Build history of the part. All positions in model axes, mm. A direction names the side the tool comes from. Round coordinates to 2 decimals unless told otherwise and drop trailing zeros. Write each loop counter-clockwise with the first axis right and the second up, starting at its lowest first coordinate (ties: lowest second). Pieces come first, ordered by that corner, then holes. Notation, with made-up numbers: (20.25, 88) -> (65.25, 88) arc R28 ccw to (65.25, 111) -> close; hole circle Ø4 at (74, 60). An arc over 180 degrees is marked (long way). Return JSON: item names as keys, results as strings.
Autodesk Inventor part; units mm, degrees
ref_plane "YZ Plane" through (0, 0, 0) normal (1, 0, 0) x (0, 1, 0)
ref_plane "XZ Plane" through (0, 0, 0) normal (0, 1, 0) x (-1, 0, 0)
ref_plane "XY Plane" through (0, 0, 0) normal (0, 0, 1) x (1, 0, 0)
sketch "Szkic1" plane through (0, 0, 0) normal (1, 0, 0) x (0, 1, 0)
  arc A0 (-13.3906, 4.8738) -> (13.3906, 4.8738) centre (0, 0) ccw
  arc A1 (-16.7323, 0.7692) -> (16.7323, 0.7692) centre (0, 0) ccw
  line L0 (13.3906, 4.8738) -> (15.7399, 5.7288)
  line L1 (0, 0) -> (16.75, 0) construction
  line L2 (0, 0) -> (0, 14)
  line L3 (-13.3906, 4.8738) -> (-15.7399, 5.7288)
  line L4 (0, 14) -> (0, 16.75)
  line L5 (12.5, 24) -> (22.5, 24)
  line L6 (-12.5, 24) -> (-22.5, 24)
  line L7 (22.2845, 26.5) -> (12.5, 26.5)
  line L8 (12.5, 26.5) -> (12.5, 24)
  line L9 (22.2845, 26.5) -> (22.2845, 28)
  line L10 (22.2845, 28) -> (12.5, 28)
  line L11 (12.5, 28) -> (12.5, 30.5)
  line L12 (12.5, 30.5) -> (22.2845, 30.5)
  line L13 (-22.5, 24) -> (-12.5, 24)
  line L14 (-12.5, 24) -> (-12.5, 26.5)
  line L15 (-12.5, 26.5) -> (-22.5, 26.5)
  line L16 (-22.5, 26.5) -> (-22.5, 28)
  line L17 (-22.5, 28) -> (-12.5, 28)
  line L18 (-12.5, 28) -> (-12.5, 30.5)
  line L19 (-12.5, 30.5) -> (-22.5, 30.5)
  line L20 (22.5, 24) -> (22.5, 8.1893)
  line L21 (22.5, 8.1893) -> (15.7399, 5.7288)
  line L22 (-22.5, 24) -> (-22.5, 8.1893)
  line L23 (-22.5, 8.1893) -> (-15.7399, 5.7288)
  line L24 (-22.5, 30.5) -> (-27.5, 30.5)
  line L25 (-27.5, 30.5) -> (-27.5, 10.0092)
  line L26 (22.2845, 30.5) -> (27.2845, 30.5)
  line L27 (27.2845, 30.5) -> (27.2845, 10.0135)
  line L28 (20.83, 2.2606) -> (27.2845, 4.6099)
  line L29 (27.2845, 4.6099) -> (27.2845, 10.0135)
  line L30 (20.83, 2.2606) -> (16.7323, 0.7692)
  line L31 (-20.83, 2.2606) -> (-16.7323, 0.7692)
  line L32 (-20.83, 2.2606) -> (-27.5, 4.6099)
  line L33 (-27.5, 4.6099) -> (-27.5, 10.0092)
  dimension "d26" = 5
  dimension "d27" = 5
extrude "Wyciągnięcie proste1" add sketch "Szkic1" along normal blind 75
sketch "Szkic2" plane through (0, 12.5, 30.5) normal (0, 0, 1) x (1, 0, 0)
  line L0 (0, 14.7845) -> (75, 14.7845)
  line L1 (0, 14.7845) -> (9, 14.7845)
  line L2 (75, -40) -> (75, -33.33)
  line L3 (75, -40) -> (66, -40)
  line L4 (9, 14.7845) -> (66, 14.7845)
  line L5 (66, 14.7845) -> (66, -40)
  line L6 (66, -40) -> (9, -40)
  line L7 (9, -40) -> (9, 14.7845)
  point P0 (0, -12.5)
  dimension "d32" = 9
  dimension "d33" = 9
extrude "Wyciągnięcie proste2" cut sketch "Szkic2" against normal blind 10.5
sketch "Szkic3" plane through (0, 12.5, 30.5) normal (0, 0, 1) x (1, 0, 0)
  line L0 (0, 0) -> (0, 9.7845)
  line L1 (5, 0) -> (0, 0)
  circle A0 centre (5, 5) radius 1.75
  line L2 (0, -25) -> (9, -25)
  line L3 (5, -25) -> (0, -25)
  circle A1 centre (5, -30) radius 1.75
  line L4 (66, -25) -> (75, -25)
  circle A2 centre (70, -30) radius 1.75
  circle A3 centre (70.1447, 5) radius 1.75
  point P0 (0, -12.5)
  dimension "d39" = 3.5
  dimension "d42" = 3.5
  dimension "d46" = 3.5
  dimension "d48" = 3.5
extrude "Wyciągnięcie proste3" cut sketch "Szkic3" against normal blind 10.5
properties part number "obejmadrążka"
Q1. Pin check, flat tips, straight feed: pin 1 Ø10 at (x, y) = (70, 18) entering from -Z; pin 2 Ø4 at (x, y) = (70.14, 17.5) entering from -Z; pin 3 Ø12 at (x, y) = (54, 7.5) entering from +Z; pin 4 Ø4 at (y, z) = (19.5, 13) entering from +X. Stop position of each tip, or through.
Verdict:
{"pin 1": "stops at z = -10.56", "pin 2": "stops at z = -6.35", "pin 3": "stops at z = 4.91", "pin 4": "passes through"}
Q2. Saw through at D-D on x = 5. Count the separate pieces of the cut face and the enclosed holes in it, then the cut area to 3 significant figures.
Verdict:
{"separate pieces": "5", "enclosed holes": "0", "area": "541 mm²"}
Q3. Wall check: L1, parallel to Y at x = 5, z = 24.9; L2, parallel to Y at x = 40.5, z = 15.5; L3, parallel to Y at x = 49, z = 0. Give the ranges that are in metal, low to high.
Verdict:
{"L1": "y = -27.5 to -19.25, -15.75 to -12.5, 12.5 to 15.75, 19.25 to 27.28", "L2": "y = -27.5 to -22.5, 22.5 to 27.28", "L3": "y = -16.75 to -14.25, 14.25 to 16.75"}
Q4. 3-axis set-ups, long thin cutter, end or side, ignore diameter. For faces 4 (the flat face through (72, 17, 24)), 5 (the flat face through (9, 21, 26)), 6 (the cylindrical face through (4.772, -15.765, 29.268)), 7 (the flat face through (4, -12.5, 25)), 8 (the flat face through (4, 20, 30.5)): which of +Z, -Z, +X, -X, +Y, -Y reach the whole face in a straight line?
Verdict:
{"face 4": "+X, -X", "face 5": "+Z, +Y, -Y", "face 6": "+Z", "face 7": "+Z, +X, -X", "face 8": "+Z, +X, -X, +Y, -Y"}
Q5. Two-plate mould, pull along Y, no slides. Class faces 1 (the flat face through (70, -20, 30.5)), 2 (the flat face through (72, 17, 26.5)), 3 (the flat face through (36.98, -24.12, 3.42)): +Y half, -Y half, draft (parallel to the pull), parting line (faces both ways), or undercut.
Verdict:
{"face 1": "draft", "face 2": "undercut", "face 3": "-Y half"}
Q6. Saw through at B-B on z = 21.5. List the corners of the cut face in (x, y), then the cut area to 3 significant figures.
Verdict:
{"outline": "(0, -27.5) -> (9, -27.5) -> (9, -22.5) -> (0, -22.5) -> close; (0, 22.5) -> (9, 22.5) -> (9, 27.28) -> (0, 27.28) -> close; (66, -27.5) -> (75, -27.5) -> (75, -22.5) -> (66, -22.5) -> close; (66, 22.5) -> (75, 22.5) -> (75, 27.28) -> (66, 27.28) -> close", "area": "176 mm²"}
Q7. Saw through at C-C on x = 20. List the corners of the cut face in (y, z).
Verdict:
{"outline": "(-27.5, 4.61) -> (-20.83, 2.26) -> (-16.73, 0.77) arc R16.75 ccw (long way) to (16.73, 0.77) -> (20.83, 2.26) -> (27.28, 4.61) -> (27.28, 20) -> (22.5, 20) -> (22.5, 8.19) -> (15.74, 5.73) -> (13.39, 4.87) arc R14.25 cw (long way) to (-13.39, 4.87) -> (-15.74, 5.73) -> (-22.5, 8.19) -> (-22.5, 20) -> (-27.5, 20) -> close"}
Q8. Saw through at A-A on z = 16.5. List the corners of the cut face in (x, y).
Verdict:
{"outline": "(0, -27.5) -> (75, -27.5) -> (75, -22.5) -> (0, -22.5) -> close; (0, 22.5) -> (75, 22.5) -> (75, 27.28) -> (0, 27.28) -> close"}
